Can you work these out from the model? Positions are in its coordinate system, mm. Round coordinates to 2 decimals unless told otherwise and drop trailing zeros. Order: outer loops, then holes, each group sorted by start corner. A loop starts at its lowest first (then second) coordinate and runs counter-clockwise, first axis right, second up. Notation, with made-up numbers: (61.5, 44) -> (82.5, 44) arc R14 cw to (82.5, 48) -> close; hole circle Ø3 at (71.5, -17). An arc over 180 degrees is marked (long way). Use a Markdown table: item, result. Add a question column.
Q1. If we section it at C-C on z = -11: List the corners of the cut face in (x, y) for me, plus the area to 3 significant figures.
Q2. I'm going to push flat-ended pins straight in: pin 1 Ø0.5 at (y, z) = (1, -16.5) entering from -X; pin 2 Ø2.5 at (x, z) = (-22.9, 3.75) entering from -Y. Where does each tip first touch, or does it pass through?
Q3. If we section it at A-A on x = -22.9: List the corners of the cut face in (y, z) for me.
Q4. If we section it at D-D on x = -37: List the corners of the cut face in (y, z) for me.
Q5. I need wall thicknesses on line 1 along X through (y, z) = (1.2, -34); line 2 along Z through (x, y) = (-22.9, 0.35); line 3 along Z through (x, y) = (-33, 1.5). Which ranges of each line are inside material? Lowest first, please. Write a range as [from, to].
Q6. If we section it at B-B on y = 0.7: List the corners of the cut face in (x, z) for me, plus the area to 3 significant figures.
Autodesk Inventor part; units mm, degrees
ref_plane "YZ Plane" through (0, 0, 0) normal (1, 0, 0) x (0, 1, 0)
ref_plane "XZ Plane" through (0, 0, 0) normal (0, 1, 0) x (-1, 0, 0)
ref_plane "XY Plane" through (0, 0, 0) normal (0, 0, 1) x (1, 0, 0)
sketch "Эскиз1" plane through (0, 0, 0) normal (0, 1, 0) x (-1, 0, 0)
  circle A0 centre (22.9, 3.75) radius 1.5
  circle A1 centre (53.2667, -35.05) radius 1.5
  circle A2 centre (22.9, -35.05) radius 1.5
  circle A3 centre (33.4, -38.2774) radius 3.3
  circle A4 centre (33.4, 6.9774) radius 3.3
  circle A5 centre (53.2667, 3.75) radius 1.5
  line L0 (63.2, -24.15) -> (51.2, -24.15)
  line L1 (51.2, -24.15) -> (51.2, -7.15)
  line L2 (51.2, -7.15) -> (63.2, -7.15)
  line L3 (63.2, -7.15) -> (63.2, 7.5)
  line L4 (63.2, 7.5) -> (46.0869, 7.5)
  arc A6 (35.969, 10.672) -> (46.0869, 7.5) centre (46.0869, 25.2227) ccw
  arc A7 (35.969, 10.672) -> (30.831, 10.672) centre (33.4, 6.9774) ccw
  arc A8 (20.7131, 7.5) -> (30.831, 10.672) centre (20.7131, 25.2227) ccw
  line L5 (20.7131, 7.5) -> (-2.1, 7.5)
  line L6 (-2.1, 7.5) -> (-2.1, -38.8)
  line L7 (-2.1, -38.8) -> (20.7131, -38.8)
  arc A9 (30.831, -41.972) -> (20.7131, -38.8) centre (20.7131, -56.5227) ccw
  arc A10 (30.831, -41.972) -> (35.969, -41.972) centre (33.4, -38.2774) ccw
  arc A11 (46.0869, -38.8) -> (35.969, -41.972) centre (46.0869, -56.5227) ccw
  line L8 (46.0869, -38.8) -> (63.2, -38.8)
  line L9 (63.2, -38.8) -> (63.2, -24.15)
  circle A12 centre (30.5522, -15.6437) radius 50
  line L10 (53.2667, -35.05) -> (22.9, -35.05)
  line L11 (53.2667, 3.75) -> (22.9, 3.75)
  point P0 (0, 0)
  point P1 (-2.1, -15.65)
  point P2 (0, 0)
  point P3 (-63.2, 38.8)
  point P4 (63.2, -38.8)
  dimension "d7" = 3.75
  dimension "d8" = 3.75
  dimension "d9" = 9.9333
  dimension "d10" = 9.9333
  dimension "d11" = 25
  dimension "d12" = 25
  dimension "d13" = 3
sketch "Эскиз2" plane through (0, 0, 0) normal (0, 1, 0) x (-1, 0, 0)
  line L0 (63.2, 7.5) -> (-2.1, 7.5)
  line L1 (-2.1, 7.5) -> (-2.1, -38.8)
  line L2 (-2.1, -38.8) -> (63.2, -38.8)
  line L3 (63.2, -38.8) -> (63.2, 7.5)
  arc A0 (35.969, 10.672) -> (46.0869, 7.5) centre (46.0869, 25.2227) ccw
  arc A1 (35.969, 10.672) -> (30.831, 10.672) centre (33.4, 6.9774) ccw
  arc A2 (20.7131, 7.5) -> (30.831, 10.672) centre (20.7131, 25.2227) ccw
  arc A3 (46.0869, -38.8) -> (35.969, -41.972) centre (46.0869, -56.5227) ccw
  arc A4 (30.831, -41.972) -> (35.969, -41.972) centre (33.4, -38.2774) ccw
  arc A5 (30.831, -41.972) -> (20.7131, -38.8) centre (20.7131, -56.5227) ccw
  arc A6 (46.0869, 7.5) -> (35.969, 4.328) centre (46.0869, -10.2227) ccw
  arc A7 (30.831, 4.328) -> (35.969, 4.328) centre (33.4, 8.0226) ccw
  arc A8 (30.831, 4.328) -> (20.7131, 7.5) centre (20.7131, -10.2227) ccw
  arc A9 (35.969, -35.628) -> (46.0869, -38.8) centre (46.0869, -21.0773) ccw
  arc A10 (35.969, -35.628) -> (30.831, -35.628) centre (33.4, -39.3226) ccw
  arc A11 (20.7131, -38.8) -> (30.831, -35.628) centre (20.7131, -21.0773) ccw
  circle A12 centre (53.2667, 3.75) radius 1.5
  circle A13 centre (53.2667, -35.05) radius 1.5
  circle A14 centre (22.9, -35.05) radius 1.5
  circle A15 centre (22.9, 3.75) radius 1.5
  line L4 (51.2, -7.15) -> (63.2, -7.15)
  line L5 (51.2, -24.15) -> (51.2, -7.15)
  line L6 (63.2, -24.15) -> (51.2, -24.15)
  line L7 (49.7, 2.1365) -> (49.6974, -33.4365)
  line L8 (5.237, 2.1365) -> (49.7, 2.1365)
  line L9 (49.6974, -33.4365) -> (5.2344, -33.4365)
  line L10 (5.2344, -33.4365) -> (5.237, 2.1365)
  circle A16 centre (33.6662, -30.3764) radius 1.397
  circle A17 centre (33.6662, -0.9236) radius 1.397
  line L11 (49.7, 2.1365) -> (49.7, -33.4365) construction
  line L12 (49.7, -15.65) -> (51.2, -15.65) construction
  arc A18 (-19.4267, 43.6888) -> (-16.3877, 43.6879) centre (-17.9094, 36.2928) ccw
  circle A19 centre (-3.0489, 41.4072) radius 1.397
  circle A20 centre (-32.5129, 41.4072) radius 1.397
  line L13 (-3.0489, 41.4072) -> (-32.5129, 41.4072)
  line L14 (-17.7809, 41.4072) -> (-17.7809, 38)
  line L15 (30.5522, -15.6437) -> (30.5522, -33.4365) construction
  line L16 (33.6662, -30.3764) -> (33.6662, -0.9236) construction
  dimension "d0" = 35.573
  dimension "d1" = 1.5
  dimension "d4" = 3.0601
  dimension "d5" = 3.0601
  dimension "d6" = 3.114
extrude "Выдавливание1" add sketch "Эскиз2" along normal blind 1.6 contours L3 L4 L5 L6 L2 A9 A10 A11 L1 L0 A8 A7 A6 | L7 L9 L10 L8
equation "\"d12\" = d11"
equation "\"d5\" = d4"
properties part number "openMV_board"
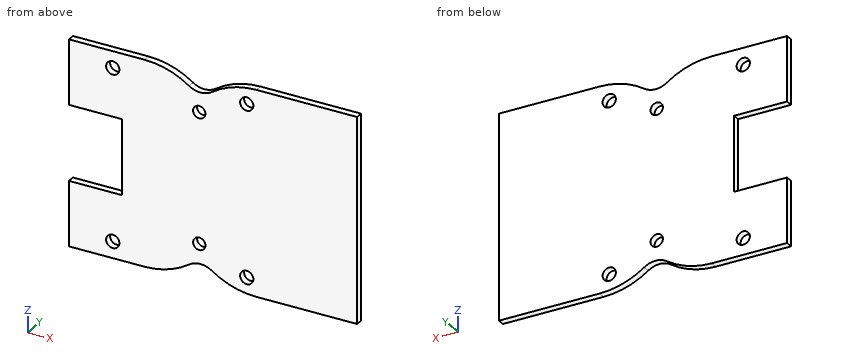
Answer below:
| question | item | result |
|---|---|---|
| 1 | outline | (-51.2, 0) -> (2.1, 0) -> (2.1, 1.6) -> (-51.2, 1.6) -> close |
| 1 | area | 85.3 mm² |
| 2 | pin 1 | x = -51.2 |
| 2 | pin 2 | through |
| 3 | outline | (0, -38.66) -> (1.6, -38.66) -> (1.6, -36.55) -> (0, -36.55) -> close; (0, -33.55) -> (1.6, -33.55) -> (1.6, 2.25) -> (0, 2.25) -> close; (0, 5.25) -> (1.6, 5.25) -> (1.6, 7.36) -> (0, 7.36) -> close |
| 4 | outline | (0, -36.29) -> (1.6, -36.29) -> (1.6, 4.99) -> (0, 4.99) -> close |
| 5 | line 1 | [-63.2, -54.34], [-52.2, -23.97], [-21.83, 2.1] |
| 5 | line 2 | [-38.66, -36.55], [-33.55, 2.25], [5.25, 7.36] |
| 5 | line 3 | [-34.84, -31.6], [-29.15, -2.15], [0.3, 3.54] |
| 6 | outline | (-63.2, -38.8) -> (-46.09, -38.8) arc R17.72 ccw to (-35.97, -35.63) arc R4.5 cw to (-30.83, -35.63) arc R17.72 ccw to (-20.71, -38.8) -> (2.1, -38.8) -> (2.1, 7.5) -> (-20.71, 7.5) arc R17.72 ccw to (-30.83, 4.33) arc R4.5 cw to (-35.97, 4.33) arc R17.72 ccw to (-46.09, 7.5) -> (-63.2, 7.5) -> (-63.2, -7.15) -> (-51.2, -7.15) -> (-51.2, -24.15) -> (-63.2, -24.15) -> close; hole circle Ø3 at (-53.27, -35.05); hole circle Ø3 at (-53.27, 3.75); hole circle Ø2.79 at (-33.67, -30.38); hole circle Ø2.79 at (-33.67, -0.92); hole circle Ø3 at (-22.9, -35.05); hole circle Ø3 at (-22.9, 3.75) |
| 6 | area | 2,700 mm² |
